Input: part model. Units: mm. Frame: model coordinates. Face numbers are marked on the shaded views. A direction names the side the tool comes from. Give positions to 0.01 mm unless a question says otherwise; leave off trailing zeros. Loops run counter-clockwise (first coordinate to the right, second up) from the corner with the lowest first, then second, coordinate; pieces in that order, holes last. Notation, with made-up numbers: (-36.75, 89.25) -> (-32.75, 89.25) arc R10 ccw to (-32.75, 107.25) -> close; hole circle Ø1 at (43.5, -7). An arc over 180 degrees is marked (long way). Answer as a JSON object with one key per item and string values. Group by question number.
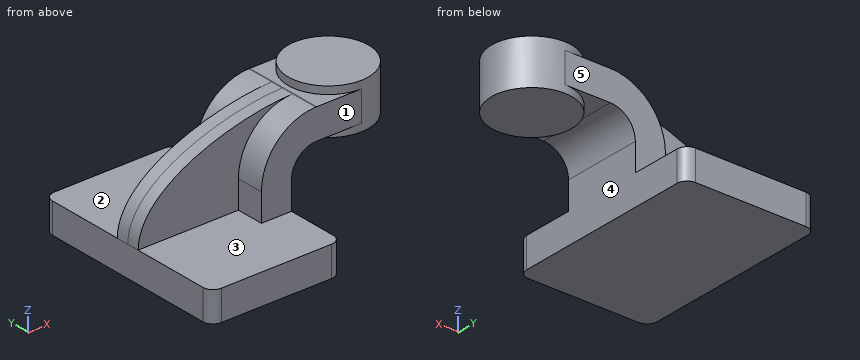
```python
from build123d import *

# Parameters (mm, degrees)
F1_DEPTH = 63.5
F0_W     = 25.4
F0_H     = 19.05
F2_DEPTH = 25.4
F3_DEPTH = 7.9375
F5_R     = 6.35


with BuildPart() as f1:
    # F0 (on Front) → F1 (new body, symmetric)
    with BuildSketch(Plane.XZ):
        Polygon((41.275, -9.525), (41.275, 9.525), (22.225, 9.525), (-41.275, 9.525), (-41.275, -9.525), align=None)
    extrude(amount=F1_DEPTH, both=True)

    # F0 (on Front) → F2 (join, symmetric)
    with BuildSketch(Plane.XZ):
        with BuildLine():
            Line((22.225, 9.525), (41.275, 9.525))
            Line((41.275, 9.525), (41.275, 27.0002))
            ThreePointArc((41.275, 27.0002), (45.9246798487, 38.2255201513), (57.15, 42.8752))
            Line((57.15, 42.8752), (60.325, 42.8752))
            Line((60.325, 42.8752), (60.325, 61.9252))
            Line((60.325, 61.9252), (57.15, 61.9252))
            add(Edge.make_bspline(
                [(56.5697529207, 61.9203795288), (56.7642060535, 61.9225634714), (56.9576279056, 61.9241702866), (57.15, 61.9252)],
                knots=[110.8594899862, 110.8594899862, 110.8594899862, 110.8594899862, 111.5045361635, 111.5045361635, 111.5045361635, 111.5045361635], degree=3))
            ThreePointArc((56.5697529207, 61.9203795288), (32.2499924273, 51.4898967698), (22.225, 27.0002))
            Line((22.225, 27.0002), (22.225, 9.525))
        make_face()
        Polygon((41.275, -9.525), (41.275, 9.525), (22.225, 9.525), (-41.275, 9.525), (-41.275, -9.525), align=None)
        with Locations((73.025, 52.4002)):
            Rectangle(F0_W, F0_H)
    extrude(amount=F2_DEPTH, both=True)

    # F0 (on Front) → F3 (join, symmetric)
    with BuildSketch(Plane.XZ):
        with BuildLine():
            Line((-41.275, 9.525), (22.225, 9.525))
            Line((22.225, 9.525), (22.225, 27.0002))
            ThreePointArc((22.225, 27.0002), (32.2499924273, 51.4898967698), (56.5697529207, 61.9203795288))
            add(Edge.make_bspline(
                [(-41.275, 9.525), (-40.7295745203, 44.1231784774), (23.1504786353, 61.5450408791), (56.5697529207, 61.9203795288)],
                knots=[0, 0, 0, 0, 110.8594899862, 110.8594899862, 110.8594899862, 110.8594899862], degree=3))
        make_face()
    extrude(amount=F3_DEPTH, both=True)

    # F0 (on Front) → F4 (revolve)
    with BuildSketch(Plane.XZ):
        Polygon((85.725, 61.9252), (85.725, 42.8752), (85.725, 38.1), (111.125, 38.1), (111.125, 66.675), (85.725, 66.675), align=None)
    revolve(axis=Axis((85.725, 0, 52.3875), (0, 0, 1)))

    # F5
    f5_edges = [f1.edges().sort_by_distance(p)[0] for p in [
        (-41.275, -63.5, 0),
        (41.275, -63.5, 0),
        (41.275, 63.5, 0),
        (-41.275, 63.5, 0),
    ]]
    fillet(f5_edges, radius=F5_R)


solid = f1.part
```
Q1. Ray query, probe 1 along Z at (x, y) = (-7, 55) (3 decimals); probe 2 along Y at (x, z) = (-28.5, 33); probe 3 along X at (y, z) = (-35, 6) (3 decimals). Return the intervals inside material, ascending.
Q2. Section A-A on y = -37. Return the cut outline in (x, z) (3 decimals), then the cut area to 3 significant figures.
Q3. Set-up query: the marked faces 1, 2, 3, 4 and 5. Return all of +Z, -Z, +X, -X, +Y, -Y with unobstructed straight access to the full face (end or side cutting, diameter ignored); none if empty.
Q4. Pin query (flat end, axial travel): pin 1 Ø18.5 at (y, z) = (22, 3.5) entering from +X (3 decimals); pin 2 Ø14 at (y, z) = (16, 19) entering from -X (3 decimals); pin 3 Ø1 at (x, z) = (-15, 37) entering from -Y. Return the tip coordinate at first contact, or that it passes through.
Q5. Section B-B on x = 73.5. Return the cut outline in (y, z) (3 decimals).
Numbers:
{
 "1": {"probe 1": "z = -9.525 to 9.525", "probe 2": "y = -7.94 to 7.94", "probe 3": "x = -41.275 to 41.275"},
 "2": {"outline": "(-41.275, -9.525) -> (41.275, -9.525) -> (41.275, 9.525) -> (-41.275, 9.525) -> close", "area": "1,570 mm²"},
 "3": {"face 1": "+Z, +X, -X, -Y", "face 2": "+Z, -X, +Y", "face 3": "+Z, -X, -Y", "face 4": "-Z, +X, +Y, -Y", "face 5": "+Z, +X, -X, +Y"},
 "4": {"pin 1": "stops at x = 41.275", "pin 2": "stops at x = 22.225", "pin 3": "stops at y = -7.94"},
 "5": {"outline": "(-25.4, 42.875) -> (-22.265, 42.875) -> (-22.265, 38.1) -> (22.265, 38.1) -> (22.265, 42.875) -> (25.4, 42.875) -> (25.4, 61.925) -> (22.265, 61.925) -> (22.265, 66.675) -> (-22.265, 66.675) -> (-22.265, 61.925) -> (-25.4, 61.925) -> close"}
}
